Could you check a few things on this drawing? It's one solid part, dimensions in mm from its lowest x, y, z. Give positions to 0.01 mm unless a question says otherwise; leave off trailing zeros. Loops run counter-clockwise (first coordinate to the right, second up) from the corner with the lowest first, then second, coordinate; pieces in that order, holes last. Notation, with made-up numbers: M 23,47.5 L 34,47.5 A10 cw 34,66.5 Z; hole C -11.5,-27.5 d8. An arc over 180 degrees is marked long. Answer as CSV lines item,"result". Start each with the question number.
Item 1: If I drill on line 1 along Z through (x, y) = (37, 1.3); line 2 along X through (y, z) = (0.25, 6.75); line 3 along X through (y, z) = (1.55, 11.5), over which ranges is the centre line in solid material (lowest first)? Write a range as from..to.
Item 2: I want a section at B-B on y = 1.45. List the corners of the cut face in (x, z) for me, plus the area to 3 significant figures.
Item 3: I want a section at A-A on x = 49. List the corners of the cut face in (y, z) for me.
Item 4: I want a section at C-C on z = 7.25. List the corners of the cut face in (x, y) for me, plus the area to 3 significant figures.
Item 5: I want a section at D-D on x = 37. List the corners of the cut face in (y, z) for me.
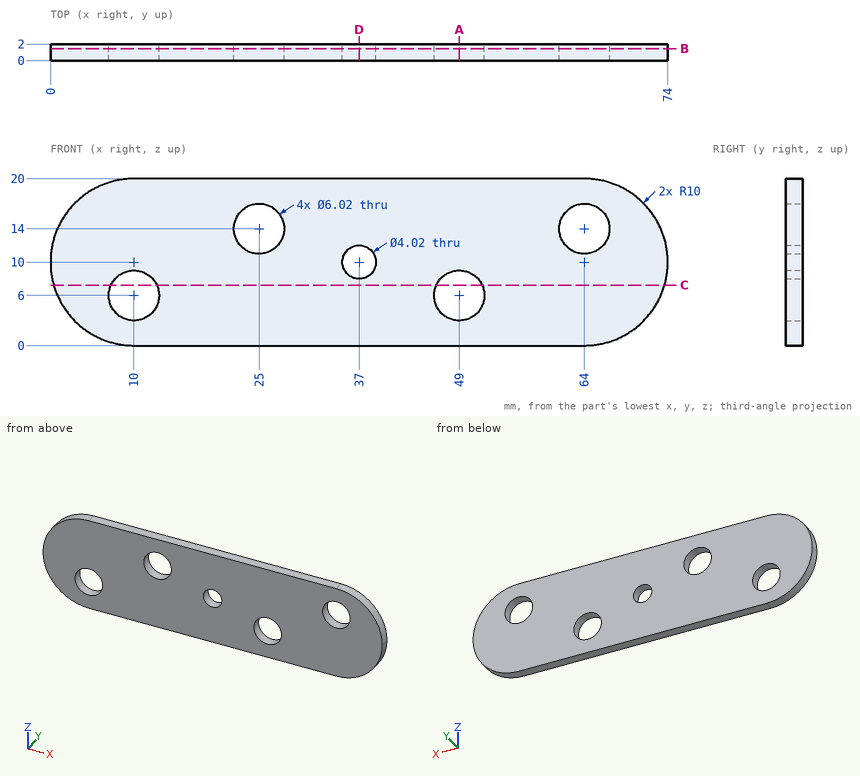
Result:
1,line 1,"0..7.99, 12.01..20"
1,line 2,"0.54..7.08, 12.92..46.08, 51.92..73.46"
1,line 3,"0.11..23.32, 26.68..35.66, 38.34..62.32, 65.68..73.89"
2,outline,"M 0,10 A10 ccw 10,0 L 64,0 A10 ccw 74,10 A10 ccw 64,20 L 10,20 A10 ccw Z; hole C 10,6 d6.02; hole C 25,14 d6.02; hole C 37,10 d4.02; hole C 49,6 d6.02; hole C 64,14 d6.02"
2,area,"1,270 mm^2"
3,outline,"M 0,0 L 2,0 L 2,2.99 L 0,2.99 Z; M 0,9.01 L 2,9.01 L 2,20 L 0,20 Z"
4,outline,"M 0.39,0 L 7.26,0 L 7.26,2 L 0.39,2 Z; M 12.74,0 L 46.26,0 L 46.26,2 L 12.74,2 Z; M 51.74,0 L 73.61,0 L 73.61,2 L 51.74,2 Z"
4,area,"125 mm^2"
5,outline,"M 0,0 L 2,0 L 2,7.99 L 0,7.99 Z; M 0,12.01 L 2,12.01 L 2,20 L 0,20 Z"
